Check sheet for the drawn part. Datum: minimum x, y, z corner. Units: mm. A direction names the side the tool comes from. Give positions to 0.01 mm unless a question says otherwise; leave off trailing zeros. Write each loop counter-clockwise with the first axis right and the second up, starting at its lowest first coordinate (ties: lowest second). Pieces come first, ordered by that corner, then holes. Notation, with made-up numbers: M 22.5,35.25 L 52.5,35.25 A11 cw 52.5,39.25 Z; hole C 72,74.5 d2. An arc over 180 degrees is marked long. Write item = value, one per line. Start each with the question number.
1) Set-up check for the marked faces 1 and 2: record each of +Z, -Z, +X, -X, +Y, -Y from which the full face is reachable in a straight line by a thin tool's end or side.
2) Scan lines: L1, parallel to X at y = 6, z = 2.25; L2, parallel to X at y = 1.75, z = 3 (1 decimal); L3, parallel to Y at x = 8.25, z = 4.5 (1 decimal). Record each from-to range of solid material in increasing order.
3) Gauge pin test, flat ends, axial feed: pin 1 (3 mm diameter, centred on x = 10.5, z = 2.5, fed in from +Y); pin 2 (2 mm diameter, centred on x = 10.5, y = 6, fed in from -Z) (1 decimal). Record the tip position at first contact, or that the pin passes through.
4) Sectioned sample at B-B, the plane x = 10.25. Record the cut outline in (y, z) (1 decimal), then the cut area to 3 significant figures.
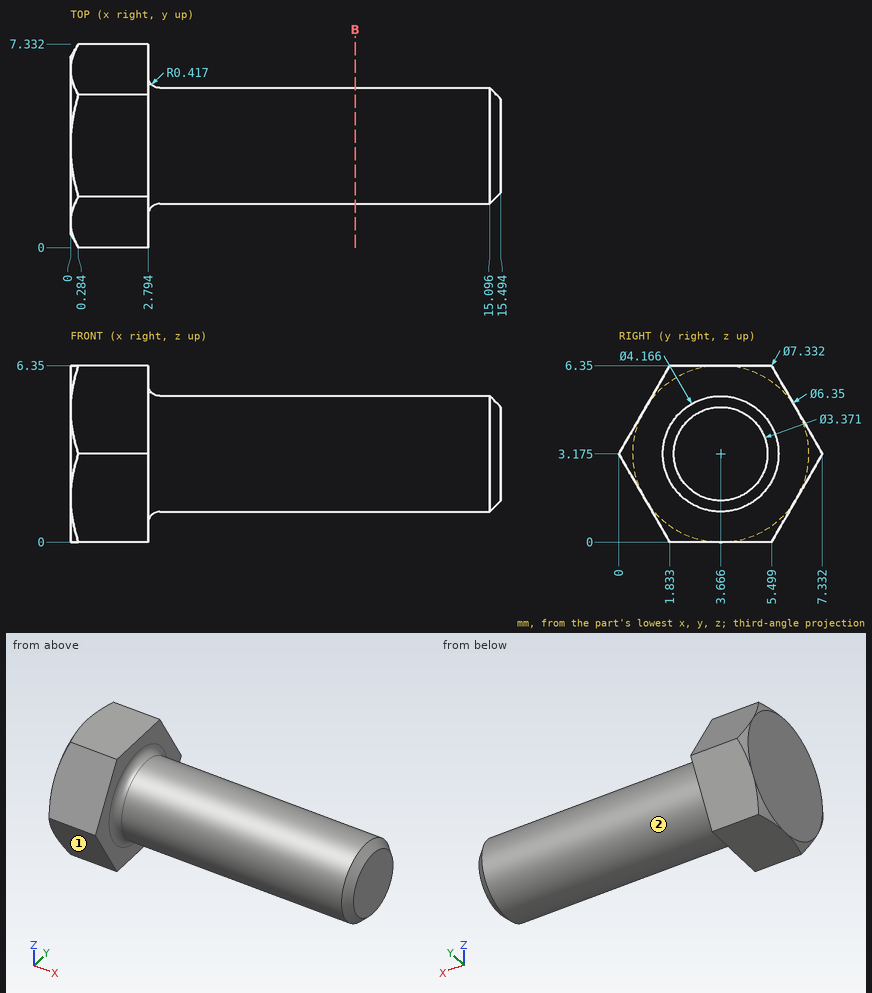
Data:
q1.face_1 = -Z, +X, -X, -Y
q1.face_2 = +X
q2.L1 = 0 to 2.79
q2.L2 = 0 to 15.3
q2.L3 = 2.1 to 5.3
q3.pin_1 = 5.75
q3.pin_2 = 1.6
q4.outline = C 3.7,3.2 d4.2
q4.area = 13.6 mm2
